Verification items for the finished model (mm, model axes). Face numbers are marked on the shaded views. Coordinates: 2 decimals unless noted, no trailing zeros. Order: outer loops, then holes, each group sorted by start corner. A loop starts at its lowest first (then second) coordinate and runs counter-clockwise, first axis right, second up.
Q1. Cross-section at B-B, the plane y = 7. Record the boundary of the cut face in (x, z), and give its area (3 significant figures).
Q2. Draft check along X on the marked faces 1, 2 and 3. Enter one of: pulls with the +X half, pulls with the -X half, needs draft (parallel to the pull), parting line crosses it, or undercut.
Q3. Thickness scan on line 1 (Y direction, x = 41.5, z = 2.25); line 2 (X direction, y = 4.75, z = 1.75); line 3 (Y direction, x = 9.5, z = 2.5). Record the ranges inside material, lowest first.
Q4. Cross-section at A-A, the plane x = 41.45. Record the boundary of the cut face in (y, z), and give its area (4 significant figures).
Q5. Depth check by flat-ended pin: P1, Ø8, axis at x = 6.5, y = 7, coming from the -Z side. Enter the tip coordinate at first touch or a pass-through.
Q6. Cross-section at C-C, the plane z = 5.5. Count the separate pieces of the cut face and the enclosed holes in it, and give its area (3 significant figures).
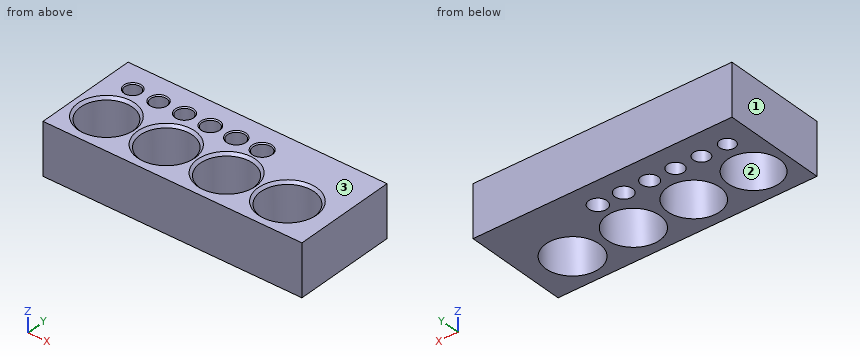
from build123d import *

# Parameters (mm, degrees)
SKETCH_W        = 50
SKETCH_H        = 20
PAD_DEPTH       = 10
SKETCH001_R     = 1.5
SKETCH001_R_2   = 1.55
SKETCH001_R_3   = 1.6
SKETCH001_R_4   = 1.7
SKETCH001_R_5   = 1.75
SKETCH001_R_6   = 1.65
SKETCH001_R_7   = 5
SKETCH001_R_8   = 5.05
SKETCH001_R_9   = 5.1
SKETCH001_R_10  = 5.15
POCKET_DEPTH    = 10.001
CHAMFER_SIZE    = 0.5
CHAMFER001_SIZE = 0.5
CHAMFER002_SIZE = 0.5
CHAMFER003_SIZE = 0.2


with BuildPart() as part:
    # Sketch → Pad (new body)
    with BuildSketch(Plane.XY):
        with Locations((25, 10)):
            Rectangle(SKETCH_W, SKETCH_H)
    extrude(amount=PAD_DEPTH)

    # Sketch001 (on Face6 of Pad) → Pocket (cut, through all)
    with BuildSketch(Plane.XY.offset(10)):
        with Locations((5, 15)):
            Circle(SKETCH001_R)
        with Locations((10, 15)):
            Circle(SKETCH001_R_2)
        with Locations((15, 15)):
            Circle(SKETCH001_R_3)
        with Locations((25, 15)):
            Circle(SKETCH001_R_4)
        with Locations((30, 15)):
            Circle(SKETCH001_R_5)
        with Locations((20, 15)):
            Circle(SKETCH001_R_6)
        with Locations((6.5, 7)):
            Circle(SKETCH001_R_7)
        with Locations((18.05, 7)):
            Circle(SKETCH001_R_8)
        with Locations((29.7, 7)):
            Circle(SKETCH001_R_9)
        with Locations((41.45, 7)):
            Circle(SKETCH001_R_10)
    extrude(amount=-POCKET_DEPTH, mode=Mode.SUBTRACT)

    # Chamfer
    chamfer_edges = [part.edges().sort_by_distance(p)[0] for p in [
        (1.5, 7, 10),
    ]]
    chamfer(chamfer_edges, length=CHAMFER_SIZE)

    # Chamfer001
    chamfer001_edges = [part.edges().sort_by_distance(p)[0] for p in [
        (13, 7, 10),
        (24.6, 7, 10),
    ]]
    chamfer(chamfer001_edges, length=CHAMFER001_SIZE)

    # Chamfer002
    chamfer002_edges = [part.edges().sort_by_distance(p)[0] for p in [
        (36.3, 7, 10),
    ]]
    chamfer(chamfer002_edges, length=CHAMFER002_SIZE)

    # Chamfer003
    chamfer003_edges = [part.edges().sort_by_distance(p)[0] for p in [
        (3.5, 15, 10),
        (8.45, 15, 10),
        (13.4, 15, 10),
        (18.35, 15, 10),
        (23.3, 15, 10),
        (28.25, 15, 10),
    ]]
    chamfer(chamfer003_edges, length=CHAMFER003_SIZE)


solid = part.part
Check values:
1. outline: (0, 0) - (1.5, 0) - (1.5, 9.5) - (1, 10) - (0, 10) - close; (11.5, 0) - (13, 0) - (13, 9.5) - (12.5, 10) - (12, 10) - (11.5, 9.5) - close; (23.1, 0) - (24.6, 0) - (24.6, 9.5) - (24.1, 10) - (23.6, 10) - (23.1, 9.5) - close; (34.8, 0) - (36.3, 0) - (36.3, 9.5) - (35.8, 10) - (35.3, 10) - (34.8, 9.5) - close; (46.6, 0) - (50, 0) - (50, 10) - (47.1, 10) - (46.6, 9.5) - close
1. area: 93.0 mm2
2. face 1: pulls with the -X half
2. face 2: undercut
2. face 3: needs draft
3. line 1: y = 0 to 1.85, 12.15 to 20
3. line 2: x = 0 to 2.03, 10.97 to 13.53, 22.57 to 25.12, 34.28 to 36.82, 46.08 to 50
3. line 3: y = 0 to 3, 11 to 13.53, 16.47 to 20
4. outline: (0, 0) - (1.85, 0) - (1.85, 9.5) - (1.35, 10) - (0, 10) - close; (12.15, 0) - (20, 0) - (20, 10) - (12.65, 10) - (12.15, 9.5) - close
4. area: 96.75 mm2
5. P1: passes through
6. separate pieces: 1
6. enclosed holes: 10
6. area: 626 mm2
